Model file for the job. Use its own axes, mm. Face numbers are marked on the shaded views. A direction names the side the tool comes from. Coordinates: 2 decimals unless noted, no trailing zeros. Write each loop counter-clockwise with the first axis right and the second up, starting at its lowest first coordinate (ties: lowest second). Pieces come first, ordered by that corner, then holes.
Q1. Pin check, flat tips, straight feed: P1, Ø5, axis at x = 0, y = 0, coming from the -Z side; P2, Ø2, axis at x = -6.5, z = 3, coming from the +Y side. Stop position of each tip, or through.
Q2. Which spindle directions (+Z, -Z, +X, -X, +Y, -Y) get a long thin tool onto all of the face, cutting with end or side? Do the marked faces 1, 2 and 3. Say none if no direction does.
Q3. Pull direction X, two halves, no side cores. Call the marked faces 4, 5 and 6: released by +X, released by -X, zero draft, split by the parting line, or undercut.
Q4. Band-saw the part on C-C, the plane z = 1.5. State how many separate pieces and enclosed holes the cut face has, plus the area to 3 significant figures.
Q5. Band-saw the part on A-A, the plane y = 0. Write the cut outline in (x, z).
Q6. Drill centre lines: probe 1 along Y at (x, z) = (0, 1.75); probe 2 along X at (y, z) = (-0.25, 0.5); probe 3 along X at (y, z) = (9, 4.5). Where is each one in solid material? Low to high.
from build123d import *

# Parameters (mm, degrees)
F0_R     = 1.6
F1_DEPTH = 6.35


with BuildPart() as f1:
    # F0 (on Top) → F1 (new body)
    with BuildSketch(Plane.XY):
        with BuildLine():
            Line((0.5, 13.107544), (-0.5, 13.107544))
            ThreePointArc((-0.5, 13.107544), (-0.764193, 12.229191), (-0.914082, 11.324295))
            ThreePointArc((-0.914082, 11.324295), (-1.482925, 11.263931), (-2.048008, 11.175011))
            ThreePointArc((-2.048008, 11.175011), (-2.426993, 12.010279), (-2.909519, 12.790325))
            Line((-2.909519, 12.790325), (-3.875445, 12.531506))
            ThreePointArc((-3.875445, 12.531506), (-3.903302, 11.614704), (-3.813879, 10.701847))
            ThreePointArc((-3.813879, 10.701847), (-4.347715, 10.496313), (-4.870529, 10.264168))
            ThreePointArc((-4.870529, 10.264168), (-5.452785, 10.972887), (-6.12076, 11.601467))
            Line((-6.12076, 11.601467), (-6.986785, 11.101467))
            ThreePointArc((-6.986785, 11.101467), (-6.776406, 10.208693), (-6.453766, 9.350086))
            ThreePointArc((-6.453766, 9.350086), (-6.916216, 9.013388), (-7.361132, 8.65384))
            ThreePointArc((-7.361132, 8.65384), (-8.106978, 9.18771), (-8.91488, 9.621987))
            Line((-8.91488, 9.621987), (-9.621987, 8.91488))
            ThreePointArc((-9.621987, 8.91488), (-9.18771, 8.106978), (-8.65384, 7.361132))
            ThreePointArc((-8.65384, 7.361132), (-9.013388, 6.916216), (-9.350086, 6.453766))
            ThreePointArc((-9.350086, 6.453766), (-10.208693, 6.776406), (-11.101467, 6.986785))
            Line((-11.101467, 6.986785), (-11.601467, 6.12076))
            ThreePointArc((-11.601467, 6.12076), (-10.972887, 5.452785), (-10.264168, 4.870529))
            ThreePointArc((-10.264168, 4.870529), (-10.496313, 4.347715), (-10.701847, 3.813879))
            ThreePointArc((-10.701847, 3.813879), (-11.614704, 3.903302), (-12.531506, 3.875445))
            Line((-12.531506, 3.875445), (-12.790325, 2.909519))
            ThreePointArc((-12.790325, 2.909519), (-12.010279, 2.426993), (-11.175011, 2.048008))
            ThreePointArc((-11.175011, 2.048008), (-11.263931, 1.482925), (-11.324295, 0.914082))
            ThreePointArc((-11.324295, 0.914082), (-12.229191, 0.764193), (-13.107544, 0.5))
            Line((-13.107544, 0.5), (-13.107544, -0.5))
            ThreePointArc((-13.107544, -0.5), (-12.229191, -0.764193), (-11.324295, -0.914082))
            ThreePointArc((-11.324295, -0.914082), (-11.263931, -1.482925), (-11.175011, -2.048008))
            ThreePointArc((-11.175011, -2.048008), (-12.010279, -2.426993), (-12.790325, -2.909519))
            Line((-12.790325, -2.909519), (-12.531506, -3.875445))
            ThreePointArc((-12.531506, -3.875445), (-11.614704, -3.903302), (-10.701847, -3.813879))
            ThreePointArc((-10.701847, -3.813879), (-10.496313, -4.347715), (-10.264168, -4.870529))
            ThreePointArc((-10.264168, -4.870529), (-10.972887, -5.452785), (-11.601467, -6.12076))
            Line((-11.601467, -6.12076), (-11.101467, -6.986785))
            ThreePointArc((-11.101467, -6.986785), (-10.208693, -6.776406), (-9.350086, -6.453766))
            ThreePointArc((-9.350086, -6.453766), (-9.013388, -6.916216), (-8.65384, -7.361132))
            ThreePointArc((-8.65384, -7.361132), (-9.18771, -8.106978), (-9.621987, -8.91488))
            Line((-9.621987, -8.91488), (-8.91488, -9.621987))
            ThreePointArc((-8.91488, -9.621987), (-8.106978, -9.18771), (-7.361132, -8.65384))
            ThreePointArc((-7.361132, -8.65384), (-6.916216, -9.013388), (-6.453766, -9.350086))
            ThreePointArc((-6.453766, -9.350086), (-6.776406, -10.208693), (-6.986785, -11.101467))
            Line((-6.986785, -11.101467), (-6.12076, -11.601467))
            ThreePointArc((-6.12076, -11.601467), (-5.452785, -10.972887), (-4.870529, -10.264168))
            ThreePointArc((-4.870529, -10.264168), (-4.347715, -10.496313), (-3.813879, -10.701847))
            ThreePointArc((-3.813879, -10.701847), (-3.903302, -11.614704), (-3.875445, -12.531506))
            Line((-3.875445, -12.531506), (-2.909519, -12.790325))
            ThreePointArc((-2.909519, -12.790325), (-2.426993, -12.010279), (-2.048008, -11.175011))
            ThreePointArc((-2.048008, -11.175011), (-1.482925, -11.263931), (-0.914082, -11.324295))
            ThreePointArc((-0.914082, -11.324295), (-0.764193, -12.229191), (-0.5, -13.107544))
            Line((-0.5, -13.107544), (0.5, -13.107544))
            ThreePointArc((0.5, -13.107544), (0.764193, -12.229191), (0.914082, -11.324295))
            ThreePointArc((0.914082, -11.324295), (1.482925, -11.263931), (2.048008, -11.175011))
            ThreePointArc((2.048008, -11.175011), (2.426993, -12.010279), (2.909519, -12.790325))
            Line((2.909519, -12.790325), (3.875445, -12.531506))
            ThreePointArc((3.875445, -12.531506), (3.903302, -11.614704), (3.813879, -10.701847))
            ThreePointArc((3.813879, -10.701847), (4.347715, -10.496313), (4.870529, -10.264168))
            ThreePointArc((4.870529, -10.264168), (5.452785, -10.972887), (6.12076, -11.601467))
            Line((6.12076, -11.601467), (6.986785, -11.101467))
            ThreePointArc((6.986785, -11.101467), (6.776406, -10.208693), (6.453766, -9.350086))
            ThreePointArc((6.453766, -9.350086), (6.916216, -9.013388), (7.361132, -8.65384))
            ThreePointArc((7.361132, -8.65384), (8.106978, -9.18771), (8.91488, -9.621987))
            Line((8.91488, -9.621987), (9.621987, -8.91488))
            ThreePointArc((9.621987, -8.91488), (9.18771, -8.106978), (8.65384, -7.361132))
            ThreePointArc((8.65384, -7.361132), (9.013388, -6.916216), (9.350086, -6.453766))
            ThreePointArc((9.350086, -6.453766), (10.208693, -6.776406), (11.101467, -6.986785))
            Line((11.101467, -6.986785), (11.601467, -6.12076))
            ThreePointArc((11.601467, -6.12076), (10.972887, -5.452785), (10.264168, -4.870529))
            ThreePointArc((10.264168, -4.870529), (10.496313, -4.347715), (10.701847, -3.813879))
            ThreePointArc((10.701847, -3.813879), (11.614704, -3.903302), (12.531506, -3.875445))
            Line((12.531506, -3.875445), (12.790325, -2.909519))
            ThreePointArc((12.790325, -2.909519), (12.010279, -2.426993), (11.175011, -2.048008))
            ThreePointArc((11.175011, -2.048008), (11.263931, -1.482925), (11.324295, -0.914082))
            ThreePointArc((11.324295, -0.914082), (12.229191, -0.764193), (13.107544, -0.5))
            Line((13.107544, -0.5), (13.107544, 0.5))
            ThreePointArc((13.107544, 0.5), (12.229191, 0.764193), (11.324295, 0.914082))
            ThreePointArc((11.324295, 0.914082), (11.263931, 1.482925), (11.175011, 2.048008))
            ThreePointArc((11.175011, 2.048008), (12.010279, 2.426993), (12.790325, 2.909519))
            Line((12.790325, 2.909519), (12.531506, 3.875445))
            ThreePointArc((12.531506, 3.875445), (11.614704, 3.903302), (10.701847, 3.813879))
            ThreePointArc((10.701847, 3.813879), (10.496313, 4.347715), (10.264168, 4.870529))
            ThreePointArc((10.264168, 4.870529), (10.972887, 5.452785), (11.601467, 6.12076))
            Line((11.601467, 6.12076), (11.101467, 6.986785))
            ThreePointArc((11.101467, 6.986785), (10.208693, 6.776406), (9.350086, 6.453766))
            ThreePointArc((9.350086, 6.453766), (9.013388, 6.916216), (8.65384, 7.361132))
            ThreePointArc((8.65384, 7.361132), (9.18771, 8.106978), (9.621987, 8.91488))
            Line((9.621987, 8.91488), (8.91488, 9.621987))
            ThreePointArc((8.91488, 9.621987), (8.106978, 9.18771), (7.361132, 8.65384))
            ThreePointArc((7.361132, 8.65384), (6.916216, 9.013388), (6.453766, 9.350086))
            ThreePointArc((6.453766, 9.350086), (6.776406, 10.208693), (6.986785, 11.101467))
            Line((6.986785, 11.101467), (6.12076, 11.601467))
            ThreePointArc((6.12076, 11.601467), (5.452785, 10.972887), (4.870529, 10.264168))
            ThreePointArc((4.870529, 10.264168), (4.347715, 10.496313), (3.813879, 10.701847))
            ThreePointArc((3.813879, 10.701847), (3.903302, 11.614704), (3.875445, 12.531506))
            Line((3.875445, 12.531506), (2.909519, 12.790325))
            ThreePointArc((2.909519, 12.790325), (2.426993, 12.010279), (2.048008, 11.175011))
            ThreePointArc((2.048008, 11.175011), (1.482925, 11.263931), (0.914082, 11.324295))
            ThreePointArc((0.914082, 11.324295), (0.764193, 12.229191), (0.5, 13.107544))
        make_face()
        with Locations((-4.879037, -4.879037)):
            Circle(F0_R, mode=Mode.SUBTRACT)
        with Locations((0, -6.9)):
            Circle(F0_R, mode=Mode.SUBTRACT)
        with Locations((4.879037, -4.879037)):
            Circle(F0_R, mode=Mode.SUBTRACT)
        with Locations((-6.9, 0)):
            Circle(F0_R, mode=Mode.SUBTRACT)
        with Locations((-4.879037, 4.879037)):
            Circle(F0_R, mode=Mode.SUBTRACT)
        Circle(F0_R, mode=Mode.SUBTRACT)
        with Locations((4.879037, 4.879037)):
            Circle(F0_R, mode=Mode.SUBTRACT)
        with Locations((6.9, 0)):
            Circle(F0_R, mode=Mode.SUBTRACT)
        with Locations((0, 6.9)):
            Circle(F0_R, mode=Mode.SUBTRACT)
    extrude(amount=F1_DEPTH)


solid = f1.part
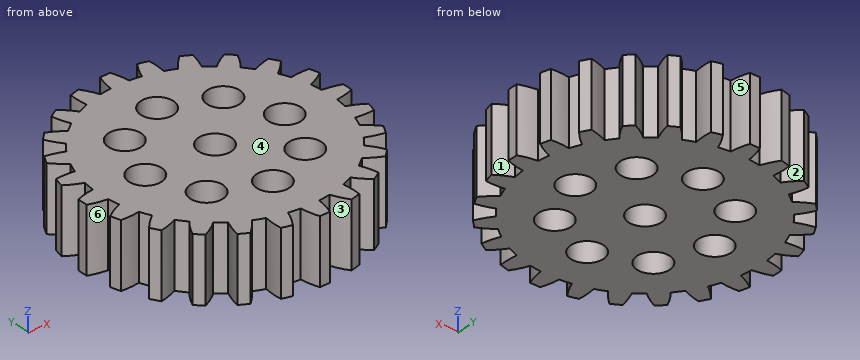
Answer sheet:
1. P1: stops at z = 0
1. P2: stops at y = 11.6
2. face 1: +Z, -Z, +X
2. face 2: +Z, -Z, +Y
2. face 3: +Z, -Z, -Y
3. face 4: zero draft
3. face 5: undercut
3. face 6: released by -X
4. separate pieces: 1
4. enclosed holes: 9
4. area: 396 mm2
5. outline: (-13.11, 0) - (-8.5, 0) - (-8.5, 6.35) - (-13.11, 6.35) - close; (-5.3, 0) - (-1.6, 0) - (-1.6, 6.35) - (-5.3, 6.35) - close; (1.6, 0) - (5.3, 0) - (5.3, 6.35) - (1.6, 6.35) - close; (8.5, 0) - (13.11, 0) - (13.11, 6.35) - (8.5, 6.35) - close
6. probe 1: y = -13.11 to -8.5, -5.3 to -1.6, 1.6 to 5.3, 8.5 to 13.11
6. probe 2: x = -13.11 to -8.48, -5.32 to -1.58, 1.58 to 5.32, 8.48 to 13.11
6. probe 3: x = -9.54 to -7.82, -6.93 to 6.93, 7.82 to 9.54
